Verification items for the finished model (mm, model axes). Give positions to 0.01 mm unless a question says otherwise; leave off trailing zeros. Loops run counter-clockwise (first coordinate to the right, second up) from the corner with the lowest first, then second, coordinate; pieces in that order, holes last. Notation, with made-up numbers: (80.25, 9.5) - (134.25, 9.5) arc R22 ccw to (134.25, 31.5) - close; hole circle Ø11 at (-14.75, 83.5). An arc over 180 degrees is marked (long way). Answer in a Markdown table with one row per item.
```python
from build123d import *

# Parameters (mm, degrees)
F0_W     = 177.8
F0_H     = 76.2
F1_DEPTH = 6.35
F3_DEPTH = 6.351


with BuildPart() as f1:
    # F0 (on Front) → F1 (new body)
    with BuildSketch(Plane.XZ):
        with Locations((88.9, -38.1)):
            Rectangle(F0_W, F0_H)
    extrude(amount=F1_DEPTH)

    # F2 (on face) → F3 (cut, through all)
    with BuildSketch(Plane.XZ.offset(6.35)):
        with BuildLine():
            ThreePointArc((50.8, -31.75), (46.309872, -33.609872), (44.45, -38.1))
            Line((44.45, -38.1), (50.8, -38.1))
            Line((50.8, -38.1), (50.8, -31.75))
        make_face()
        with BuildLine():
            ThreePointArc((127, -31.75), (122.509872, -33.609872), (120.65, -38.1))
            Line((120.65, -38.1), (127, -38.1))
            Line((127, -38.1), (127, -31.75))
        make_face()
        with BuildLine():
            Line((127, -38.1), (120.65, -38.1))
            ThreePointArc((120.65, -38.1), (122.509872, -42.590128), (127, -44.45))
            Line((127, -44.45), (127, -38.1))
        make_face()
        with BuildLine():
            Line((50.8, -38.1), (44.45, -38.1))
            ThreePointArc((44.45, -38.1), (46.309872, -42.590128), (50.8, -44.45))
            Line((50.8, -44.45), (50.8, -38.1))
        make_face()
        with BuildLine():
            Line((50.8, -31.75), (50.8, -38.1))
            Line((50.8, -38.1), (57.15, -38.1))
            ThreePointArc((57.15, -38.1), (55.290128, -33.609872), (50.8, -31.75))
        make_face()
        with BuildLine():
            Line((57.15, -38.1), (50.8, -38.1))
            Line((50.8, -38.1), (50.8, -44.45))
            ThreePointArc((50.8, -44.45), (55.290128, -42.590128), (57.15, -38.1))
        make_face()
        with BuildLine():
            Line((127, -31.75), (127, -38.1))
            Line((127, -38.1), (133.35, -38.1))
            ThreePointArc((133.35, -38.1), (131.490128, -33.609872), (127, -31.75))
        make_face()
        with BuildLine():
            Line((133.35, -38.1), (127, -38.1))
            Line((127, -38.1), (127, -44.45))
            ThreePointArc((127, -44.45), (131.490128, -42.590128), (133.35, -38.1))
        make_face()
    extrude(amount=-F3_DEPTH, mode=Mode.SUBTRACT)


solid = f1.part
```
Q1. Thickness scan on line 1 (X direction, y = -0.5, z = -38); line 2 (X direction, y = -4.25, z = -34); line 3 (Z direction, x = 129, y = -3.25). Record the ranges inside material, lowest first.
Completed:
| item | result |
|---|---|
| line 1 | 0 to 44.45, 57.15 to 120.65, 133.35 to 177.8 |
| line 2 | 0 to 45.95, 55.65 to 122.15, 131.85 to 177.8 |
| line 3 | -76.2 to -44.13, -32.07 to 0 |
Q2. Sectioned sample at B-B (z = -41). Record the cut outline in (x, y), and give its area (3 significant figures).
Completed:
| item | result |
|---|---|
| outline | (0, -6.35) - (45.15, -6.35) - (45.15, 0) - (0, 0) - close; (56.45, -6.35) - (121.35, -6.35) - (121.35, 0) - (56.45, 0) - close; (132.65, -6.35) - (177.8, -6.35) - (177.8, 0) - (132.65, 0) - close |
| area | 986 mm^2 |
Q3. Sectioned sample at A-A (y = -4.75). Record the cut outline in (x, z), and give its area (3 significant figures).
Completed:
| item | result |
|---|---|
| outline | (0, -76.2) - (177.8, -76.2) - (177.8, 0) - (0, 0) - close; hole circle Ø12.7 at (50.8, -38.1); hole circle Ø12.7 at (127, -38.1) |
| area | 13,300 mm^2 |
